Answer from the drawing. Dimensions are ordinates in mm from the lowest x, y and z of the part. A direction names the side the tool comes from. Give positions to 0.01 mm unless a question says otherwise; leave off trailing zeros. Loops run counter-clockwise (first coordinate to the right, second up) from the corner with the lowest first, then second, coordinate; pieces in that order, holes last. Notation, with made-up numbers: (27.25, 37.5) - (84.25, 37.5) arc R15 cw to (84.25, 65.5) - close; hole circle Ø2 at (16, -2.5). An arc over 180 degrees is marked (long way). Write each question's results on one line, items separated by ' | '. Start each with the question number.
Q1. Determine the mould class of the marked faces 1, 2, 3 and 4 for opening direction X: +X half, -X half, draft (parallel to the pull), parting line (faces both ways), or undercut.
Q2. For the marked faces 5 and 6, determine the directions among +Z, -Z, +X, -X, +Y, -Y from which every point of the face is accessible in a straight line to the end or side of a thin tool.
Q3. Given pin 1 (6 mm diameter, centred on x = 46, y = 13, fed in from -Z); pin 2 (6 mm diameter, centred on x = 33.5, z = 2.5, fed in from +Y); pin 3 (5 mm diameter, centred on y = 29, z = 5.75, fed in from -X); pin 4 (6 mm diameter, centred on y = 29.5, z = 10, fed in from -X), each flat-ended and moving along its own axis, determine where each tip first touches the part or whether it passes through.
Q4. Find the intervals of material crossed by line 1 (Z direction, x = 52, y = 29); line 2 (X direction, y = 23, z = 10.5); line 3 (Y direction, x = 51.8, z = 5.75), in increasing order. Write a range as from..to.
Q5. The part is cut by section C-C, the plane y = 17. Write down the section's boundary in (x, z).
Q6. The part is cut by section B-B, the plane z = 8. Write down the section's boundary in (x, y), plus the area to 4 significant figures.
Q7. The part is cut by section A-A, the plane y = 29. Write down the section's boundary in (x, z), plus the area to 3 significant figures.
Q8. The part is cut by section D-D, the plane x = 51. Write down the section's boundary in (y, z).
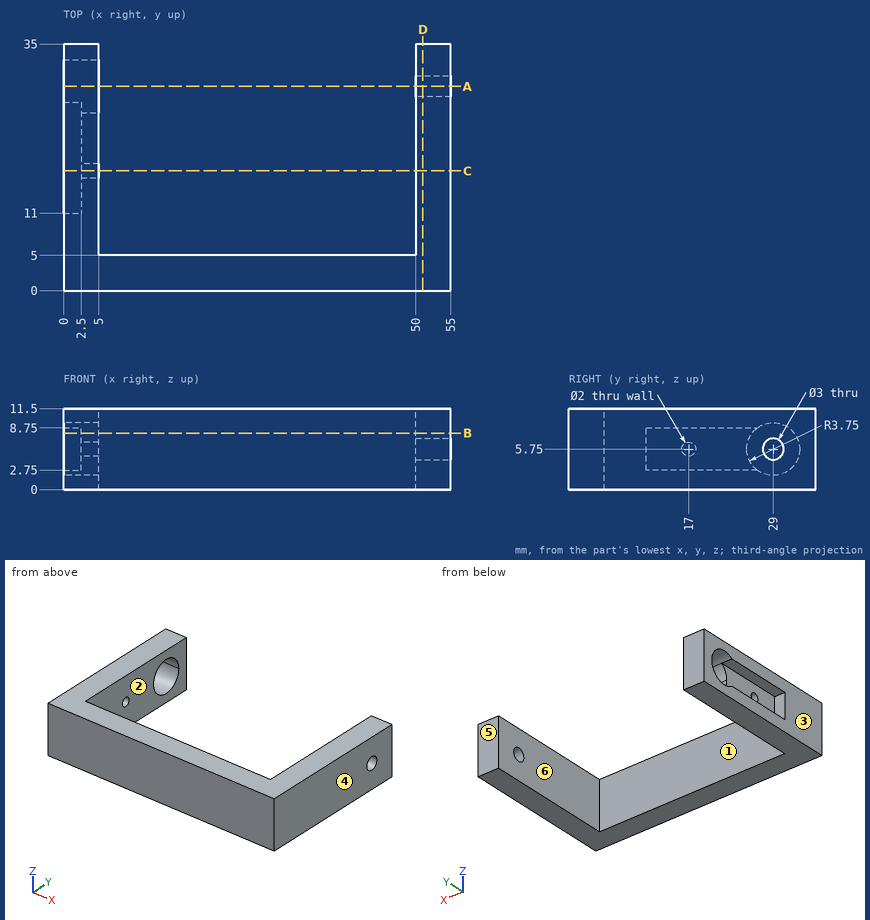
Check sheet entries:
1) face 1: undercut | face 2: undercut | face 3: -X half | face 4: +X half
2) face 5: +Z, -Z, +X, -X, +Y | face 6: +Z, -Z, +Y
3) pin 1: passes through | pin 2: stops at y = 5 | pin 3: stops at x = 50 | pin 4: stops at x = 0
4) line 1: z = 0..4.25, 7.25..11.5 | line 2: x = 0..5, 50..55 | line 3: y = 0..27.5, 30.5..35
5) outline: (0, 0) - (5, 0) - (5, 4.75) - (2.5, 4.75) - (2.5, 2.75) - (0, 2.75) - close; (0, 8.75) - (2.5, 8.75) - (2.5, 6.75) - (5, 6.75) - (5, 11.5) - (0, 11.5) - close; (50, 0) - (55, 0) - (55, 11.5) - (50, 11.5) - close
6) outline: (0, 0) - (55, 0) - (55, 35) - (50, 35) - (50, 5) - (5, 5) - (5, 26) - (2.5, 26) - (2.5, 11) - (0, 11) - close; (0, 32) - (5, 32) - (5, 35) - (0, 35) - close | area: 507.5 mm^2
7) outline: (0, 0) - (5, 0) - (5, 2) - (0, 2) - close; (0, 9.5) - (5, 9.5) - (5, 11.5) - (0, 11.5) - close; (50, 0) - (55, 0) - (55, 4.25) - (50, 4.25) - close; (50, 7.25) - (55, 7.25) - (55, 11.5) - (50, 11.5) - close | area: 62.5 mm^2
8) outline: (0, 0) - (35, 0) - (35, 11.5) - (0, 11.5) - close; hole circle Ø3 at (29, 5.75)
